Can you work these out from the model? Positions are in its coordinate system, mm. Face numbers are marked on the shaded views. A direction names the side the tool comes from. Give positions to 0.01 mm unless a question says otherwise; leave off trailing zeros. Write each loop counter-clockwise with the first axis right and the second up, starting at its lowest first coordinate (ties: lowest second). Pieces come first, ordered by that corner, then holes.
1. I'm going to push flat-ended pins straight in: pin 1 (1 mm diameter, centred on x = 82, y = 25, fed in from -Z) (3 decimals); pin 2 (2 mm diameter, centred on x = 82.55, y = 25.4, fed in from +Z); pin 3 (4 mm diameter, centred on x = 11.43, y = 39.37, fed in from -Z). Where does each tip first touch, or does it pass through?
2. Suppose I cut it at D-D (z = 4.75). Please give me the cut outline in (x, y).
3. Suppose I cut it at A-A (y = 6.35). Please give me the cut outline in (x, z).
4. Thinking about a two-plate mould opening in Y: for the marked faces 1 and 2, which applies, pulls with the +Y half, pulls with the -Y half, needs draft (parallel to the pull), parting line crosses it, or undercut?
5. On a 3-axis mill with a long thin cutter (end or side, diameter ignored), from which of +Z, -Z, +X, -X, +Y, -Y can I reach the whole of each face in a straight line? I mean the marked faces 3, 4 and 5. Say none if no direction works.
6. If I drill on probe 1 along X at (y, z) = (25.5, 4.5); probe 2 along X at (y, z) = (25.4, 1.2); probe 3 along Y at (x, z) = (95.25, 4.5), over which ranges is the centre line in solid material (lowest first)?
7. Suppose I cut it at C-C (y = 21). Please give me the cut outline in (x, z).
8. Suppose I cut it at B-B (x = 51). Please give me the cut outline in (y, z), and give its area (3 significant figures).
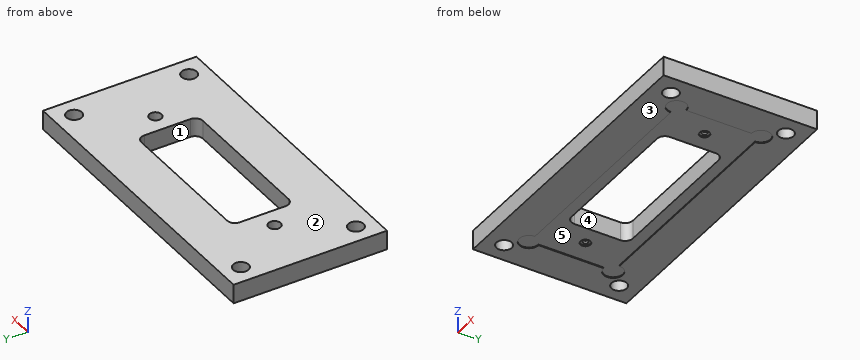
```python
from build123d import *

# Parameters (mm, degrees)
F0_W           = 101.6
F0_H           = 50.8
F1_DEPTH       = 6.35
F3_DEPTH       = 0.254
F5_DEPTH       = 25.4
F5_DEPTH_BACK  = 25.4
F6_R           = 1.651
F7_DEPTH       = 0.381
F8_R           = 2.032
F9_DEPTH       = 4.826
F10_R          = 0.8255
F11_DEPTH      = 25.4
F11_DEPTH_BACK = 5.716
F12_R          = 2.54
F13_DEPTH      = 6.351


with BuildPart() as f1:
    # F0 (on Top) → F1 (new body)
    with BuildSketch(Plane.XY):
        with Locations((50.8, 25.4)):
            Rectangle(F0_W, F0_H)
    extrude(amount=F1_DEPTH)

    # F2 (on face) → F3 (cut)
    with BuildSketch(Plane(origin=(0, 0, 0), x_dir=(1, 0, 0), z_dir=(0, 0, -1))):
        with BuildLine():
            Line((11.43, -14.605), (11.43, -11.43))
            Line((11.43, -11.43), (14.605, -11.43))
            ThreePointArc((14.605, -11.43), (9.1849359697, -9.1849359697), (11.43, -14.605))
        make_face()
        with BuildLine():
            Line((14.605, -11.43), (11.43, -11.43))
            Line((11.43, -11.43), (11.43, -14.605))
            ThreePointArc((11.43, -14.605), (13.6750640303, -13.6750640303), (14.605, -11.43))
        make_face()
        with BuildLine():
            Line((86.995, -11.43), (14.605, -11.43))
            ThreePointArc((14.605, -11.43), (13.6750640303, -13.6750640303), (11.43, -14.605))
            Line((11.43, -14.605), (11.43, -36.195))
            ThreePointArc((11.43, -36.195), (13.6750640303, -37.1249359697), (14.605, -39.37))
            Line((14.605, -39.37), (86.995, -39.37))
            ThreePointArc((86.995, -39.37), (87.9249359697, -37.1249359697), (90.17, -36.195))
            Line((90.17, -36.195), (90.17, -14.605))
            ThreePointArc((90.17, -14.605), (87.9249359697, -13.6750640303), (86.995, -11.43))
        make_face()
        with BuildLine():
            ThreePointArc((93.345, -11.43), (90.17, -8.255), (86.995, -11.43))
            Line((86.995, -11.43), (90.17, -11.43))
            Line((90.17, -11.43), (90.17, -14.605))
            ThreePointArc((90.17, -14.605), (92.4150640303, -13.6750640303), (93.345, -11.43))
        make_face()
        with BuildLine():
            Line((90.17, -11.43), (86.995, -11.43))
            ThreePointArc((86.995, -11.43), (87.9249359697, -13.6750640303), (90.17, -14.605))
            Line((90.17, -14.605), (90.17, -11.43))
        make_face()
        with BuildLine():
            ThreePointArc((14.605, -39.37), (13.6750640303, -37.1249359697), (11.43, -36.195))
            Line((11.43, -36.195), (11.43, -39.37))
            Line((11.43, -39.37), (14.605, -39.37))
        make_face()
        with BuildLine():
            Line((11.43, -39.37), (11.43, -36.195))
            ThreePointArc((11.43, -36.195), (9.1849359697, -41.6150640303), (14.605, -39.37))
            Line((14.605, -39.37), (11.43, -39.37))
        make_face()
        with BuildLine():
            ThreePointArc((93.345, -39.37), (92.4150640303, -37.1249359697), (90.17, -36.195))
            Line((90.17, -36.195), (90.17, -39.37))
            Line((90.17, -39.37), (86.995, -39.37))
            ThreePointArc((86.995, -39.37), (90.17, -42.545), (93.345, -39.37))
        make_face()
        with BuildLine():
            Line((90.17, -39.37), (90.17, -36.195))
            ThreePointArc((90.17, -36.195), (87.9249359697, -37.1249359697), (86.995, -39.37))
            Line((86.995, -39.37), (90.17, -39.37))
        make_face()
    extrude(amount=-F3_DEPTH, mode=Mode.SUBTRACT)

    # F4 (on face) → F5 (cut, two sides)
    with BuildSketch(Plane(origin=(0, 0, 0.254), x_dir=(1, 0, 0), z_dir=(0, 0, -1))) as f5_sk:
        with BuildLine():
            ThreePointArc((25.4, -33.02), (26.1439487758, -34.8160512242), (27.94, -35.56))
            Line((27.94, -35.56), (73.66, -35.56))
            ThreePointArc((73.66, -35.56), (75.4560512242, -34.8160512242), (76.2, -33.02))
            Line((76.2, -33.02), (76.2, -17.78))
            ThreePointArc((76.2, -17.78), (75.4560512242, -15.9839487758), (73.66, -15.24))
            Line((73.66, -15.24), (27.94, -15.24))
            ThreePointArc((27.94, -15.24), (26.1439487758, -15.9839487758), (25.4, -17.78))
            Line((25.4, -17.78), (25.4, -33.02))
        make_face()
    extrude(amount=F5_DEPTH, mode=Mode.SUBTRACT)
    extrude(f5_sk.sketch, amount=-F5_DEPTH_BACK, mode=Mode.SUBTRACT)

    # F6 (on face) → F7 (cut)
    with BuildSketch(Plane(origin=(0, 0, 0.254), x_dir=(1, 0, 0), z_dir=(0, 0, -1))):
        with Locations((82.55, -25.4)):
            Circle(F6_R)
        with Locations((19.05, -25.4)):
            Circle(F6_R)
    extrude(amount=-F7_DEPTH, mode=Mode.SUBTRACT)

    # F8 (on face) → F9 (cut)
    with BuildSketch(Plane.XY.offset(6.35)):
        with Locations((19.05, 25.4)):
            Circle(F8_R)
        with Locations((82.55, 25.4)):
            Circle(F8_R)
    extrude(amount=-F9_DEPTH, mode=Mode.SUBTRACT)

    # F10 (on face) → F11 (cut, two sides)
    with BuildSketch(Plane(origin=(0, 0, 0.635), x_dir=(1, 0, 0), z_dir=(0, 0, -1))) as f11_sk:
        with Locations((19.05, -25.4)):
            Circle(F10_R)
        with Locations((82.55, -25.4)):
            Circle(F10_R)
    extrude(amount=F11_DEPTH, mode=Mode.SUBTRACT)
    extrude(f11_sk.sketch, amount=-F11_DEPTH_BACK, mode=Mode.SUBTRACT)

    # F12 (on face) → F13 (cut, through all)
    with BuildSketch(Plane(origin=(0, 0, 0), x_dir=(1, 0, 0), z_dir=(0, 0, -1))):
        with Locations((95.25, -6.35)):
            Circle(F12_R)
        with Locations((6.35, -6.35)):
            Circle(F12_R)
        with Locations((6.35, -44.45)):
            Circle(F12_R)
        with Locations((95.25, -44.45)):
            Circle(F12_R)
    extrude(amount=-F13_DEPTH, mode=Mode.SUBTRACT)


solid = f1.part
```
Checks:
1. pin 1: stops at z = 0.635
1. pin 2: stops at z = 1.52
1. pin 3: stops at z = 0.25
2. outline: (0, 0) - (101.6, 0) - (101.6, 50.8) - (0, 50.8) - close; hole circle Ø5.08 at (6.35, 6.35); hole circle Ø5.08 at (6.35, 44.45); hole circle Ø4.06 at (19.05, 25.4); hole (25.4, 17.78) arc R2.54 ccw to (27.94, 15.24) - (73.66, 15.24) arc R2.54 ccw to (76.2, 17.78) - (76.2, 33.02) arc R2.54 ccw to (73.66, 35.56) - (27.94, 35.56) arc R2.54 ccw to (25.4, 33.02) - close; hole circle Ø4.06 at (82.55, 25.4); hole circle Ø5.08 at (95.25, 6.35); hole circle Ø5.08 at (95.25, 44.45)
3. outline: (0, 0) - (3.81, 0) - (3.81, 6.35) - (0, 6.35) - close; (8.89, 0) - (92.71, 0) - (92.71, 6.35) - (8.89, 6.35) - close; (97.79, 0) - (101.6, 0) - (101.6, 6.35) - (97.79, 6.35) - close
4. face 1: undercut
4. face 2: needs draft
5. face 3: -Z, +X, -X, +Y, -Y
5. face 4: +Z, -Z
5. face 5: -Z
6. probe 1: x = 0 to 17.02, 21.08 to 25.4, 76.2 to 80.52, 84.58 to 101.6
6. probe 2: x = 0 to 18.22, 19.88 to 25.4, 76.2 to 81.72, 83.38 to 101.6
6. probe 3: y = 0 to 3.81, 8.89 to 41.91, 46.99 to 50.8
7. outline: (0, 0) - (11.43, 0) - (11.43, 0.25) - (25.4, 0.25) - (25.4, 6.35) - (0, 6.35) - close; (76.2, 0.25) - (90.17, 0.25) - (90.17, 0) - (101.6, 0) - (101.6, 6.35) - (76.2, 6.35) - close
8. outline: (0, 0) - (11.43, 0) - (11.43, 0.25) - (15.24, 0.25) - (15.24, 6.35) - (0, 6.35) - close; (35.56, 0.25) - (39.37, 0.25) - (39.37, 0) - (50.8, 0) - (50.8, 6.35) - (35.56, 6.35) - close
8. area: 192 mm2
